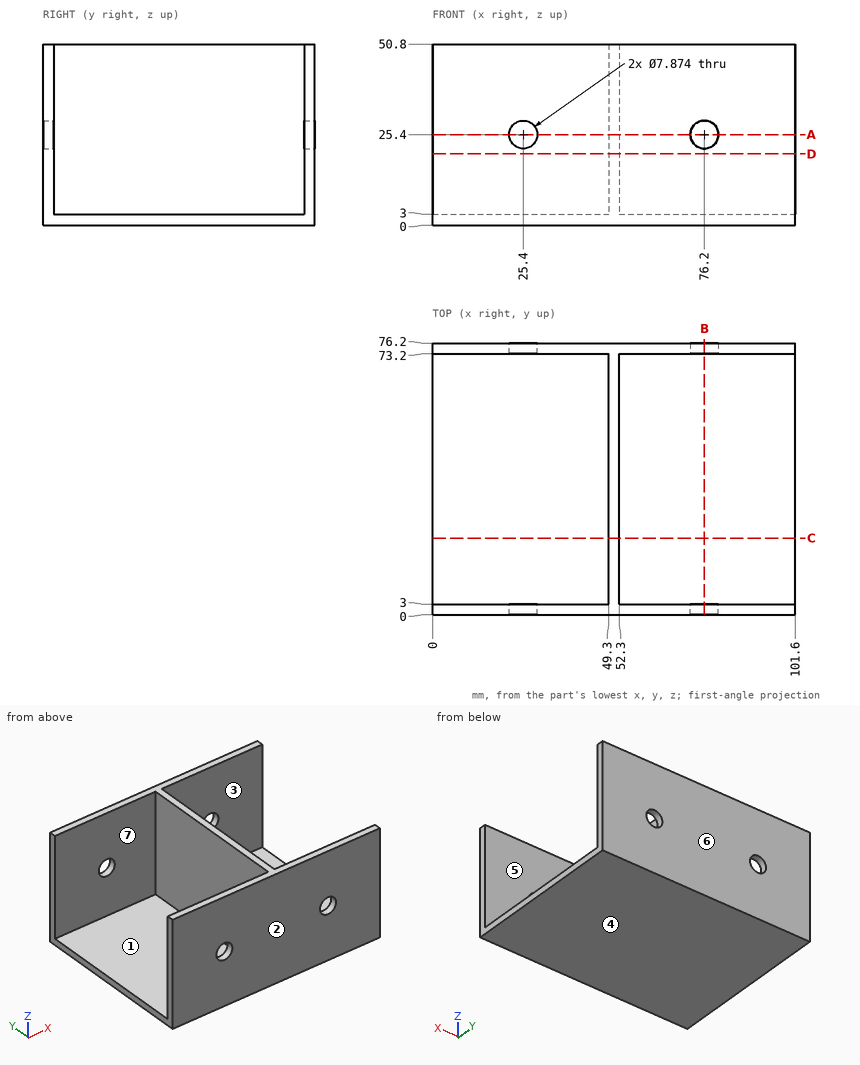
Design review of the part shown in the three views and the two pictorial views. Dimensions are in mm from the part's minimum x, y and z. A direction names the side the tool comes from. Give positions to 0.01 mm unless a question says otherwise; leave off trailing zeros. Loops run counter-clockwise (first coordinate to the right, second up) from the corner with the lowest first, then second, coordinate; pieces in that order, holes last. Notation, with made-up numbers: (80.5, 68.5) - (125.5, 68.5) arc R11 ccw to (125.5, 84.5) - close; hole circle Ø4 at (77.5, -39). An arc over 180 degrees is marked (long way). Write item = value, one per line.
1) Draft analysis for pull direction Y (two halves, no side actions). For the marked faces 1, 2, 3 and 4, state which applies: +Y half, -Y half, draft (parallel to the pull), parting line (faces both ways), or undercut.
Result sheet:
face_1 = undercut
face_2 = -Y half
face_3 = undercut
face_4 = draft
2) Tool access review of the marked faces 5, 6 and 7: name each direction out of +Z, -Z, +X, -X, +Y, -Y from which nothing blocks a thin tool from reaching the whole face with its end or side.
Result sheet:
face_5 = +Z, +X
face_6 = +Z, -Z, +X, -X, +Y
face_7 = +Z, -X
3) Take a section at B-B on x = 76.2. State the section outline as (y, z) points, and give its area (3 significant figures).
Result sheet:
outline = (0, 0) - (76.2, 0) - (76.2, 21.46) - (73.2, 21.46) - (73.2, 3) - (3, 3) - (3, 21.46) - (0, 21.46) - close; (0, 29.34) - (3, 29.34) - (3, 50.8) - (0, 50.8) - close; (73.2, 29.34) - (76.2, 29.34) - (76.2, 50.8) - (73.2, 50.8) - close
area = 468 mm2
4) Take a section at C-C on y = 21.5. State the section outline as (x, z) points, and give its area (3 significant figures).
Result sheet:
outline = (0, 0) - (101.6, 0) - (101.6, 3) - (52.3, 3) - (52.3, 50.8) - (49.3, 50.8) - (49.3, 3) - (0, 3) - close
area = 448 mm2
5) To check wall thickness, follow line 1 (X direction, y = 74.4, z = 25.4); line 2 (Y direction, x = 40, z = 16); line 3 (Z direction, x = 76.2, y = 75.6). State the ranges of each line that lie inside material, in increasing order.
Result sheet:
line_1 = 0 to 21.46, 29.34 to 72.26, 80.14 to 101.6
line_2 = 0 to 3, 73.2 to 76.2
line_3 = 0 to 21.46, 29.34 to 50.8
6) Take a section at A-A on z = 25.4. State the section outline as (x, y) points.
Result sheet:
outline = (0, 0) - (21.46, 0) - (21.46, 3) - (0, 3) - close; (0, 73.2) - (21.46, 73.2) - (21.46, 76.2) - (0, 76.2) - close; (29.34, 0) - (72.26, 0) - (72.26, 3) - (52.3, 3) - (52.3, 73.2) - (72.26, 73.2) - (72.26, 76.2) - (29.34, 76.2) - (29.34, 73.2) - (49.3, 73.2) - (49.3, 3) - (29.34, 3) - close; (80.14, 0) - (101.6, 0) - (101.6, 3) - (80.14, 3) - close; (80.14, 73.2) - (101.6, 73.2) - (101.6, 76.2) - (80.14, 76.2) - close
7) Clearance check with flat-ended pins moving along their axes: pin 1 Ø6 at (y, z) = (65, 25) entering from -X; pin 2 Ø5 at (x, z) = (50, 12.5) entering from -Y; pin 3 Ø15 at (x, y) = (13, 32.5) entering from +Z. State where each tip first meets the part, or that it passes through.
Result sheet:
pin_1 = 49.3
pin_2 = 0
pin_3 = 3
8) Take a section at D-D on z = 20. State the section outline as (x, y) points, and give its area (3 significant figures).
Result sheet:
outline = (0, 0) - (101.6, 0) - (101.6, 3) - (52.3, 3) - (52.3, 73.2) - (101.6, 73.2) - (101.6, 76.2) - (0, 76.2) - (0, 73.2) - (49.3, 73.2) - (49.3, 3) - (0, 3) - close
area = 820 mm2
